```python
from build123d import *
from build123d.topology import SkipClean

# Parameters (mm, degrees)
BOSS_EXTRUDE1_DEPTH = 27.60218
SKETCH3_R           = 7.1
SKETCH3_R_2         = 5.1
BOSS_EXTRUDE2_DEPTH = 5
SKETCH4_R           = 6.6
SKETCH4_R_2         = 5.6
BOSS_EXTRUDE3_DEPTH = 7.62
CUT_EXTRUDE1_START  = -7.62
SKETCH5_R           = 5.6
CUT_EXTRUDE1_DEPTH  = 7.62
SKETCH6_R           = 5.1
CUT_EXTRUDE2_DEPTH  = 19.05


with BuildPart() as part:
    # Sketch1 → Boss-Extrude1 (new body)
    with BuildSketch(Plane(origin=(0, 0, 0), x_dir=(0, 0, -1), z_dir=(1, 0, 0))):
        Polygon((-11.058823529, 7.635882353), (-11.058823529, -5.294117647), (0.941176471, -5.294117647), (0.941176471, -4.294117647), (-10.058823529, -4.294117647), (-10.058823529, 7.635882353), align=None)
    extrude(amount=BOSS_EXTRUDE1_DEPTH)

    # Sketch3 → Boss-Extrude2 (add)
    with BuildSketch(Plane(origin=(0, -7.176470588, 7.176470588), x_dir=(-1, 0, 0), z_dir=(0, 0.7071067811865465, -0.7071067811865487))):
        with Locations(Location((-13.80109, 4.076262621, 0), (0, 0, 90))):
            Circle(SKETCH3_R)
        with Locations(Location((-13.80109, 4.076262621, 0), (0, 0, 90))):
            Circle(SKETCH3_R_2, mode=Mode.SUBTRACT)
    extrude(amount=-BOSS_EXTRUDE2_DEPTH)

    # Sketch4 → Boss-Extrude3 (add)
    with BuildSketch(Plane(origin=(0, -7.176470588, 7.176470588), x_dir=(-1, 0, 0), z_dir=(0, 0.7071067811865465, -0.7071067811865487))):
        with Locations(Location((-13.80109, 4.076262621, 0), (0, 0, 180))):
            Circle(SKETCH4_R)
        with Locations(Location((-13.80109, 4.076262621, 0), (0, 0, 180))):
            Circle(SKETCH4_R_2, mode=Mode.SUBTRACT)
    extrude(amount=BOSS_EXTRUDE3_DEPTH)

    # Sketch5 → Cut-Extrude1 (cut)
    with SkipClean():  # the faces are left unmerged after this step: merging them gives an invalid solid
        with BuildSketch(Plane(origin=(0, -1.788316916, 1.788316916), x_dir=(1, 0, 0), z_dir=(0, 0.7071067811865465, -0.7071067811865486)).offset(CUT_EXTRUDE1_START)):
            with Locations(Location((13.80109, -4.076262621, 0), (0, 0, 270))):
                Circle(SKETCH5_R)
        extrude(amount=CUT_EXTRUDE1_DEPTH, mode=Mode.SUBTRACT)

    # Sketch6 → Cut-Extrude2 (cut)
    with SkipClean():  # the faces are left unmerged after this step: merging them gives an invalid solid
        with BuildSketch(Plane(origin=(0, -1.788316916, 1.788316916), x_dir=(1, 0, 0), z_dir=(0, 0.7071067811865465, -0.7071067811865486))):
            with Locations(Location((13.80109, -4.076262621, 0), (0, 0, 270))):
                Circle(SKETCH6_R)
        extrude(amount=-CUT_EXTRUDE2_DEPTH, mode=Mode.SUBTRACT)


solid = part.part
```
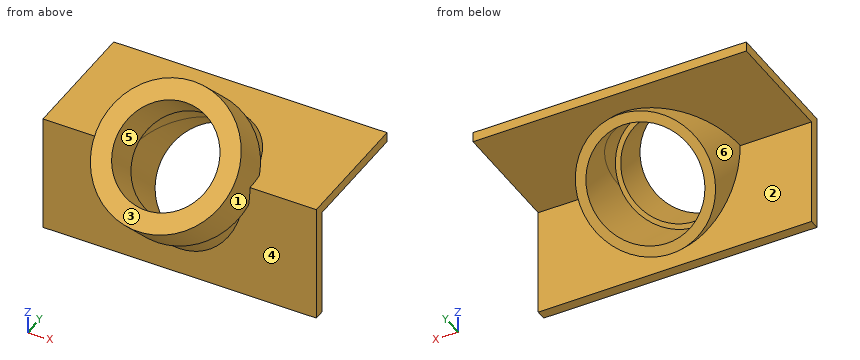
Check sheet for the modelled part. Datum: model origin and axes. Units: mm. Face numbers are marked on the shaded views. A direction names the side the tool comes from. Give positions to 0.01 mm unless a question says otherwise; leave off trailing zeros. Write each loop counter-clockwise with the first axis right and the second up, starting at its lowest first coordinate (ties: lowest second). Pieces come first, ordered by that corner, then holes. Notation, with made-up numbers: (-4, 16.5) - (44, 16.5) arc R21 cw to (44, 54.5) - close; hole circle Ø6 at (50.25, 45.25). An arc over 180 degrees is marked (long way). Answer as a JSON object with one key per item and string values. Group by question number.
1) Sectioned sample at A-A (x = 12.25). Record the cut outline in (y, z).
2) Release check for a two-part mould opening along Z. For the marked faces 3, 4, 5 and 6 record: pulls with the +Z half, pulls with the -Z half, needs draft (parallel to the pull), parting line crosses it, or undercut.
3) Access from +Z, -Z, +X, -X, +Y, -Y to the whole of each face (thin tool, end or side, straight path). Record for the marked faces 1 and 2.
4) Depth check by flat-ended pin: P1, Ø4, axis at x = 15.5, z = 4.5, coming from the +Y side; P2, Ø4, axis at y = -9.5, z = 7, coming from the +X side; P3, Ø5, axis at x = 3, z = 4, coming from the +Y side. Enter the tip coordinate at first touch or a pass-through.
5) Thickness scan on probe 1 along X at (y, z) = (-5.25, 9.75); probe 2 along X at (y, z) = (-4.5, 16.75); probe 3 along Z at (x, y) = (3.5, 2.5). Record the ranges inside material, lowest first. Write a range as from..to.
6) Sectioned sample at B-B (x = 5). Record the cut outline in (y, z).
Geometry results:
{
 "1": {"outline": "(-12.73, 8.7) - (-9.19, 5.16) - (-8.83, 5.52) - (-5.29, 1.99) - (-5.29, -0.94) - (-4.29, -0.94) - (-4.29, 0.99) - (-3.44, 0.13) - (-2.71, 0.87) - (-8.1, 6.25) - (-7.73, 6.62) - (-11.27, 10.16) - close; (-4.39, 17.03) - (-0.86, 13.49) - (-0.49, 13.86) - (4.9, 8.48) - (5.63, 9.21) - (4.78, 10.06) - (7.64, 10.06) - (7.64, 11.06) - (3.78, 11.06) - (0.24, 14.6) - (0.61, 14.96) - (-2.93, 18.49) - close"},
 "2": {"face 3": "pulls with the +Z half", "face 4": "needs draft", "face 5": "undercut", "face 6": "undercut"},
 "3": {"face 1": "none", "face 2": "-Z"},
 "4": {"P1": "stops at y = -3.9", "P2": "stops at x = 19.77", "P3": "stops at y = -4.29"},
 "5": {"probe 1": "x = 0..8.78, 18.82..27.6", "probe 2": "x = 8.38..11.57, 16.03..19.22", "probe 3": "z = 10.06..11.06"},
 "6": {"outline": "(-5.29, -0.94) - (-4.29, -0.94) - (-4.29, 10.06) - (7.64, 10.06) - (7.64, 11.06) - (-5.29, 11.06) - close"}
}
